```python
from build123d import *

# Parameters (mm, degrees)
SKETCH1_W                      = 20
SKETCH1_H                      = 26
SKETCH1_W_2                    = 1.25
SKETCH1_H_2                    = 15
BOSS_EXTRUDE5_DEPTH            = 5
SKETCH3_W                      = 7
SKETCH3_H                      = 26
BOSS_EXTRUDE6_DEPTH            = 40
CUT_EXTRUDE1_REACH             = 55.696
SKETCH5_R                      = 11.2
SKETCH6_W                      = 26
SKETCH6_H                      = 5
BOSS_EXTRUDE8_DEPTH            = 14
SKETCH8_R                      = 12
SKETCH8_R_2                    = 7.5
BOSS_EXTRUDE9_DEPTH            = 2.5
SKETCH9_R                      = 12
SKETCH9_R_2                    = 7.5
BOSS_EXTRUDE10_DEPTH           = 2.5
SKETCH7_W                      = 12
SKETCH7_H                      = 1.25
CUT_EXTRUDE2_DEPTH             = 10
BOSS_EXTRUDE11_DEPTH           = 37.12
SKETCH14_R                     = 2.25
SKETCH14_R_2                   = 4.5
CUT_EXTRUDE4_DEPTH             = 10
CUT_EXTRUDE5_REACH             = 85.48
CUT_EXTRUDE5_DIRECTION_2_REACH = 85.48


with BuildPart() as part:
    # Sketch1 → Boss-Extrude5 (new body)
    with BuildSketch(Plane(origin=(0, 0, 0), x_dir=(1, 0, 0), z_dir=(0, 1, 0))):
        with Locations((10, 13)):
            Rectangle(SKETCH1_W, SKETCH1_H)
        with Locations((1.875, 13)):
            Rectangle(SKETCH1_W_2, SKETCH1_H_2, mode=Mode.SUBTRACT)
    boss_extrude5 = extrude(amount=BOSS_EXTRUDE5_DEPTH)

    # Sketch3 → Boss-Extrude6 (add)
    with BuildSketch(Plane(origin=(0, 5, 0), x_dir=(1, 0, 0), z_dir=(0, 1, 0))):
        with Locations((10, 13)):
            Rectangle(SKETCH3_W, SKETCH3_H)
    boss_extrude6 = extrude(amount=BOSS_EXTRUDE6_DEPTH)

    # Sketch5 → Cut-Extrude1 (cut, up to next)
    with BuildSketch(Plane(origin=(13.5, 0, 0), x_dir=(0, 0, -1), z_dir=(1, 0, 0)), mode=Mode.PRIVATE) as cut_extrude1_sk1:
        with Locations((13, 20)):
            Circle(SKETCH5_R)
    cut_extrude1_tool1 = extrude(cut_extrude1_sk1.sketch, amount=-CUT_EXTRUDE1_REACH, mode=Mode.PRIVATE) & part.part
    # Sketch5 → Cut-Extrude1 (cut, up to next)
    with BuildSketch(Plane(origin=(13.5, 0, 0), x_dir=(0, 0, -1), z_dir=(1, 0, 0)), mode=Mode.PRIVATE) as cut_extrude1_sk2:
        with BuildLine():
            Line((0, 27.483314774), (0, 45))
            Line((0, 45), (26, 45))
            Line((26, 45), (26, 27.483314774))
            ThreePointArc((26, 27.483314774), (13, 35), (0, 27.483314774))
        make_face()
    cut_extrude1_tool2 = extrude(cut_extrude1_sk2.sketch, amount=-CUT_EXTRUDE1_REACH, mode=Mode.PRIVATE) & part.part
    cut_extrude1_1 = cut_extrude1_tool1.solids().sort_by_distance((13.5, 20, -13))[0]
    add(cut_extrude1_1, mode=Mode.SUBTRACT)
    cut_extrude1_2 = cut_extrude1_tool2.solids().sort_by_distance((13.5, 38.725293, -13))[0]
    add(cut_extrude1_2, mode=Mode.SUBTRACT)
    cut_extrude1 = cut_extrude1_1 + cut_extrude1_2  # Cut-Extrude1 as one shape, for the pattern or mirror that repeats it

    # Sketch6 → Boss-Extrude8 (add)
    with BuildSketch(Plane(origin=(20, 0, 0), x_dir=(0, 0, -1), z_dir=(1, 0, 0))):
        with Locations((13, 2.5)):
            Rectangle(SKETCH6_W, SKETCH6_H)
    boss_extrude8 = extrude(amount=BOSS_EXTRUDE8_DEPTH)

    # Mirror5: Boss-Extrude5, Boss-Extrude6, Cut-Extrude1, Boss-Extrude8 across plane
    add(boss_extrude5.mirror(Plane.ZY.offset(-34)))
    add(boss_extrude6.mirror(Plane.ZY.offset(-34)))
    add(cut_extrude1.mirror(Plane.ZY.offset(-34)), mode=Mode.SUBTRACT)
    add(boss_extrude8.mirror(Plane.ZY.offset(-34)))

    # Sketch8 → Boss-Extrude9 (add)
    with BuildSketch(Plane.ZY.offset(-6.5)):
        with Locations(Location((-13, 20, 0), (0, 0, 180))):
            Circle(SKETCH8_R)
        with Locations((-13, 20)):
            Circle(SKETCH8_R_2, mode=Mode.SUBTRACT)
    extrude(amount=BOSS_EXTRUDE9_DEPTH)

    # Sketch9 → Boss-Extrude10 (add)
    with BuildSketch(Plane.ZY.offset(-54.5)):
        with Locations(Location((-13, 20, 0), (0, 0, 180))):
            Circle(SKETCH9_R)
        with Locations((-13, 20)):
            Circle(SKETCH9_R_2, mode=Mode.SUBTRACT)
    extrude(amount=BOSS_EXTRUDE10_DEPTH)

    # Sketch7 → Cut-Extrude2 (cut)
    with BuildSketch(Plane(origin=(0, 5, 0), x_dir=(1, 0, 0), z_dir=(0, 1, 0))):
        with Locations((22, 1.875)):
            Rectangle(SKETCH7_W, SKETCH7_H)
        with Locations((46, 1.875)):
            Rectangle(SKETCH7_W, SKETCH7_H)
        with Locations((46, 24.125)):
            Rectangle(SKETCH7_W, SKETCH7_H)
        with Locations((22, 24.125)):
            Rectangle(SKETCH7_W, SKETCH7_H)
    extrude(amount=-CUT_EXTRUDE2_DEPTH, mode=Mode.SUBTRACT)

    # Sketch10 → Boss-Extrude11 (add)
    with BuildSketch(Plane.XY):
        Polygon((51, 0), (68, 0), (68, 5), (61.5, 5), (61.5, 47.8), (57.5, 47.8), (57.5, 5), (51, 5), align=None)
    extrude(amount=BOSS_EXTRUDE11_DEPTH)

    # Sketch14 → Cut-Extrude4 (cut)
    with BuildSketch(Plane(origin=(61.5, 0, 0), x_dir=(0, 0, -1), z_dir=(1, 0, 0))):
        Polygon((-37.12, 51.83243557), (-37.12, 47.8), (-18.56, 47.8), (0, 47.8), (0, 51.83243557), align=None)
        with BuildLine():
            Line((0, 47.8), (-18.56, 47.8))
            ThreePointArc((-18.56, 47.8), (-8.484558377, 45.75747818), (0, 39.952421039))
            Line((0, 39.952421039), (0, 47.8))
        make_face()
        with BuildLine():
            Line((-37.12, 47.8), (-37.12, 39.952421039))
            ThreePointArc((-37.12, 39.952421039), (-28.635441623, 45.75747818), (-18.56, 47.8))
            Line((-18.56, 47.8), (-37.12, 47.8))
        make_face()
        with Locations((-18.556883399, 43.896979327)):
            Circle(SKETCH14_R)
        with Locations((-10.556883399, 26.396979327)):
            Circle(SKETCH14_R_2)
        with Locations((-18.556883399, 8.896979327)):
            Circle(SKETCH14_R)
    extrude(amount=-CUT_EXTRUDE4_DEPTH, mode=Mode.SUBTRACT)

    # Cut-Extrude5: up to this face of the body (flat: up to its plane)
    cut_extrude5_end = Plane(part.part.faces().sort_by_distance((68, 2.5, 5.56))[0])
    # Sketch15 → Cut-Extrude5 (cut, up to the picked face)
    with BuildSketch(Plane.ZY.offset(-57.5), mode=Mode.PRIVATE) as cut_extrude5_sk1:
        with BuildLine():
            Line((37.12, 0), (37.12, 5))
            Line((37.12, 5), (37.12, 39.952421039))
            ThreePointArc((37.12, 39.952421039), (30.226412362, 45.020265293), (22.056883399, 47.562585579))
            Line((22.056883399, 47.562585579), (22.056883399, 0))
            Line((22.056883399, 0), (37.12, 0))
        make_face()
    cut_extrude5_tool1 = split(extrude(cut_extrude5_sk1.sketch, amount=-CUT_EXTRUDE5_REACH, mode=Mode.PRIVATE), bisect_by=cut_extrude5_end, keep=Keep.BOTH, mode=Mode.PRIVATE)
    # Sketch15 → Cut-Extrude5 (cut, up to the picked face)
    with BuildSketch(Plane.ZY.offset(-57.5), mode=Mode.PRIVATE) as cut_extrude5_sk2:
        with BuildLine():
            Line((0, 39.952421039), (0, 27.483314774))
            Line((0, 27.483314774), (15.056883399, 47.561734504))
            ThreePointArc((15.056883399, 47.561734504), (6.890780172, 45.018846696), (0, 39.952421039))
        make_face()
    cut_extrude5_tool2 = split(extrude(cut_extrude5_sk2.sketch, amount=-CUT_EXTRUDE5_REACH, mode=Mode.PRIVATE), bisect_by=cut_extrude5_end, keep=Keep.BOTH, mode=Mode.PRIVATE)
    add(cut_extrude5_tool1.solids().sort_by(Axis((57.5, 22.463316, 29.381371), (1, 0, 0)))[0], mode=Mode.SUBTRACT)
    add(cut_extrude5_tool2.solids().sort_by(Axis((57.5, 39.195611, 5.346979), (1, 0, 0)))[0], mode=Mode.SUBTRACT)

    # Cut-Extrude5 direction 2: up to this face of the body (flat: up to its plane)
    cut_extrude5_direction_2_end = Plane(part.part.faces().sort_by_distance((51, 2.5, 18.56))[0])
    # Sketch15 → Cut-Extrude5 direction 2 (cut, up to the picked face)
    with BuildSketch(Plane.ZY.offset(-57.5), mode=Mode.PRIVATE) as cut_extrude5_direction_2_sk1:
        with BuildLine():
            Line((37.12, 0), (37.12, 5))
            Line((37.12, 5), (37.12, 39.952421039))
            ThreePointArc((37.12, 39.952421039), (30.226412362, 45.020265293), (22.056883399, 47.562585579))
            Line((22.056883399, 47.562585579), (22.056883399, 0))
            Line((22.056883399, 0), (37.12, 0))
        make_face()
    cut_extrude5_direction_2_tool1 = split(extrude(cut_extrude5_direction_2_sk1.sketch, amount=CUT_EXTRUDE5_DIRECTION_2_REACH, mode=Mode.PRIVATE), bisect_by=cut_extrude5_direction_2_end, keep=Keep.BOTH, mode=Mode.PRIVATE)
    # Sketch15 → Cut-Extrude5 direction 2 (cut, up to the picked face)
    with BuildSketch(Plane.ZY.offset(-57.5), mode=Mode.PRIVATE) as cut_extrude5_direction_2_sk2:
        with BuildLine():
            Line((0, 39.952421039), (0, 27.483314774))
            Line((0, 27.483314774), (15.056883399, 47.561734504))
            ThreePointArc((15.056883399, 47.561734504), (6.890780172, 45.018846696), (0, 39.952421039))
        make_face()
    cut_extrude5_direction_2_tool2 = split(extrude(cut_extrude5_direction_2_sk2.sketch, amount=CUT_EXTRUDE5_DIRECTION_2_REACH, mode=Mode.PRIVATE), bisect_by=cut_extrude5_direction_2_end, keep=Keep.BOTH, mode=Mode.PRIVATE)
    add(cut_extrude5_direction_2_tool1.solids().sort_by(Axis((57.5, 22.463316, 29.381371), (-1, 0, 0)))[0], mode=Mode.SUBTRACT)
    add(cut_extrude5_direction_2_tool2.solids().sort_by(Axis((57.5, 39.195611, 5.346979), (-1, 0, 0)))[0], mode=Mode.SUBTRACT)


solid = part.part
```
Here's how the part is built. I have some questions about the finished solid (model axes, mm). A direction names the side the tool comes from. Coordinates: 2 decimals unless noted, no trailing zeros. Order: outer loops, then holes, each group sorted by start corner. A loop starts at its lowest first (then second) coordinate and runs counter-clockwise, first axis right, second up.
1) Imagine slicing it at D-D on z = 2.5. List the corners of the cut face in (x, y) for me, and give its area (3 significant figures).
2) I need wall thicknesses on line 1 (Y direction, x = 61, z = 18.5); line 2 (Z direction, x = 42.5, y = 4); line 3 (X direction, y = 3.5, z = -6.5). Which ranges of each line are inside material? Lowest first, please.
3) Which directions (+Z, -Z, +X, -X, +Y, -Y) give clear straight access to the entire face, cutting with the end or side of a thin tool? Please do faces 1 (the face through (6.5, 27.3, -15.3)), 2 (the face through (54.5, 27.3, -15.3)), 3 (the face through (1.25, 2, -13)), 4 (the face through (52, 25, -7)), 5 (the face through (56, 16, 0)).
4) We'd pull the mould along Z, two halves only. Please class faces 6 (the face through (41, 0, -8)), 7 (the face through (59.53, 41.7, 19.04)), 8 (the face through (34, 4, -26)): +Z half, -Z half, draft (parallel to the pull), parting line (faces both ways), or undercut.
5) Will these pins go through, and if not, where does the flat tip stop? pin 1 (8 mm diameter, centred on y = 18, z = -13, fed in from -X); pin 2 (12 mm diameter, centred on x = 26, z = -8.5, fed in from +Y); pin 3 (5 mm diameter, centred on x = 2.5, z = -12, fed in from +Y); pin 4 (12 mm diameter, centred on y = 13, z = 5, fed in from +X).
6) Imagine slicing it at C-C on x = 36. List the corners of the cut face in (y, z) for me.
7) Imagine slicing it at A-A on y = 20. State how many separate pieces and enclosed holes the cut face has, and give its area (3 significant figures).
Response values:
1. outline: (51, 0) - (68, 0) - (68, 5) - (61.5, 5) - (61.5, 30.82) - (57.5, 30.82) - (57.5, 5) - (51, 5) - close
1. area: 188 mm2
2. line 1: y = 0 to 6.65, 11.15 to 41.65, 46.15 to 47.8
2. line 2: z = -26 to -24.75, -23.5 to -2.5, -1.25 to 0
2. line 3: x = 0 to 1.25, 2.5 to 65.5, 66.75 to 68
3. face 1: none
3. face 2: +X
3. face 3: +Y, -Y
3. face 4: +Z, -Z, +Y
3. face 5: +Z, -X, +Y
4. face 6: draft
4. face 7: undercut
4. face 8: -Z half
5. pin 1: passes through
5. pin 2: stops at y = 5
5. pin 3: stops at y = 32
5. pin 4: stops at x = 61.5
6. outline: (0, -26) - (5, -26) - (5, 0) - (0, 0) - close
7. separate pieces: 4
7. enclosed holes: 0
7. area: 184 mm2
